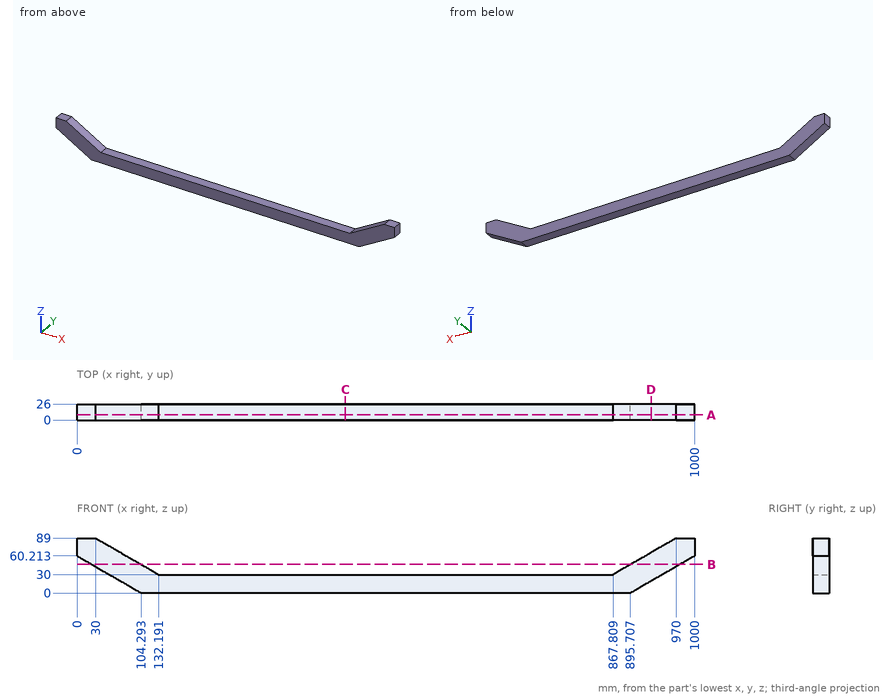
Here's the drawing with two shaded views (mm, measured from the low corner). I have some questions. Coordinates: 2 decimals unless noted, no trailing zeros. Loops run counter-clockwise (first coordinate to the right, second up) from the corner with the lowest first, then second, coordinate; pieces in that order, holes last. Notation, with made-up numbers: (42.25, 38) -> (62.25, 38) arc R22 ccw to (62.25, 66) -> close; hole circle Ø10 at (77.25, -32.5). An arc over 180 degrees is marked (long way). Answer as a JSON object with one key per item and string values.
1) Imagine slicing it at A-A (y = 8.5). Please give me the cut outline in (x, z).
Results:
{"outline": "(0, 60.21) -> (104.29, 0) -> (895.71, 0) -> (1000, 60.21) -> (1000, 89) -> (970, 89) -> (867.81, 30) -> (132.19, 30) -> (30, 89) -> (0, 89) -> close"}
2) Imagine slicing it at C-C (x = 434.5). Please give me the cut outline in (y, z).
Results:
{"outline": "(0, 0) -> (26, 0) -> (26, 30) -> (0, 30) -> close"}
3) Imagine slicing it at B-B (z = 46.5). Please give me the cut outline in (x, y), then the cut area to 3 significant figures.
Results:
{"outline": "(23.75, 0) -> (103.61, 0) -> (103.61, 26) -> (23.75, 26) -> close; (896.39, 0) -> (976.25, 0) -> (976.25, 26) -> (896.39, 26) -> close", "area": "4,150 mm^2"}
4) For P1, Ø3, axis at x = 632.5, y = 14, coming from the -Z side; P2, Ø5, axis at x = 197, y = 13.5, coming from the +Z side; P3, Ø1, axis at y = 5.5, z = 38.5, coming from the +X side (1 decimal), each with a flat end and sliding along its axis, tell me the tip position at first contact or that it passes through.
Results:
{"P1": "stops at z = 0", "P2": "stops at z = 30", "P3": "stops at x = 963.3"}
5) Imagine slicing it at D-D (x = 929). Please give me the cut outline in (y, z), then the cut area to 3 significant figures.
Results:
{"outline": "(0, 19.22) -> (26, 19.22) -> (26, 65.33) -> (0, 65.33) -> close", "area": "1,200 mm^2"}
6) If I drill on line 1 (Z direction, x = 212.5, y = 5.25); line 2 (X direction, y = 1.25, z = 70); line 3 (X direction, y = 20.5, z = 84), over which ranges is the centre line in solid material (lowest first)?
Results:
{"line 1": "z = 0 to 30", "line 2": "x = 0 to 62.91, 937.09 to 1000", "line 3": "x = 0 to 38.66, 961.34 to 1000"}
